CAD build for the part. Positions are in the model's coordinates, mm. A direction names the side the tool comes from. Give positions to 0.01 mm unless a question says otherwise; leave off trailing zeros. Write each loop counter-clockwise with the first axis right and the second up, starting at its lowest first coordinate (ties: lowest second). Pieces come first, ordered by that corner, then holes. Notation, with made-up numbers: (-12.5, 73) - (-7.5, 73) arc R21 cw to (-7.5, 83) - close; hole circle Ø2 at (41, -36.75). An arc over 180 degrees is marked (long way). Answer as a JSON object with one key per item and string values.
from build123d import *

# Parameters (mm, degrees)
SKETCH1_R               = 19.05
BASE_EXTRUDE_DEPTH      = 47.625
CUT_EXTRUDE1_DEPTH      = 20.05
CUT_EXTRUDE1_DEPTH_BACK = 20.05
CUT_EXTRUDE5_DEPTH      = 20.0500001
CUT_EXTRUDE5_DEPTH_BACK = 20.0500001
SKETCH11_R              = 4.7625
CUT_EXTRUDE6_DEPTH      = 20.0500001
CUT_EXTRUDE6_DEPTH_BACK = 20.0500001
SKETCH12_R              = 4.7625
CUT_EXTRUDE7_DEPTH      = 48.625000104
SCALE1_SCALE            = 0.65


with BuildPart() as part:
    # Sketch1 → Base-Extrude (new body)
    with BuildSketch(Plane(origin=(0, 0, 0), x_dir=(-1, 0, 0), z_dir=(0, 1, 0))):
        Circle(SKETCH1_R)
    extrude(amount=BASE_EXTRUDE_DEPTH)

    # Sketch2 → Cut-Extrude1 (cut, two sides)
    with BuildSketch(Plane.XY) as cut_extrude1_sk:
        with BuildLine():
            Line((-19.05, -131.979516723), (-19.05, 0))
            Line((-19.05, 0), (-19.05, 29.21))
            ThreePointArc((-19.05, 29.21), (-12.314807909, 26.420192091), (-9.525, 19.685))
            Line((-9.525, 19.685), (-9.525, 9.525))
            ThreePointArc((-9.525, 9.525), (0, 0), (9.525, 9.525))
            Line((9.525, 9.525), (9.525, 19.685))
            ThreePointArc((9.525, 19.685), (12.314807909, 26.420192091), (19.05, 29.21))
            Line((19.05, 29.21), (19.05, 0))
            Line((19.05, 0), (19.05, -131.979516723))
            Line((19.05, -131.979516723), (19.05, -395.938550169))
            Line((19.05, -395.938550169), (-19.05, -395.938550169))
            Line((-19.05, -395.938550169), (-19.05, -131.979516723))
        make_face()
    extrude(amount=CUT_EXTRUDE1_DEPTH, mode=Mode.SUBTRACT)
    extrude(cut_extrude1_sk.sketch, amount=-CUT_EXTRUDE1_DEPTH_BACK, mode=Mode.SUBTRACT)

    # Sketch8 → Cut-Extrude5 (cut, two sides)
    with BuildSketch(Plane(origin=(0, 0, 0), x_dir=(0, 0, -1), z_dir=(1, 0, 0))) as cut_extrude5_sk:
        Polygon((-10.16, -121.738350451), (-10.16, 0), (-10.16, 29.145238826), (10.16, 29.145238826), (10.16, 0), (10.16, -121.738350451), (10.16, -365.215051352), (-10.16, -365.215051352), align=None)
    extrude(amount=CUT_EXTRUDE5_DEPTH, mode=Mode.SUBTRACT)
    extrude(cut_extrude5_sk.sketch, amount=-CUT_EXTRUDE5_DEPTH_BACK, mode=Mode.SUBTRACT)

    # Sketch11 → Cut-Extrude6 (cut, two sides)
    with BuildSketch(Plane.XY) as cut_extrude6_sk:
        with Locations((0, 9.525)):
            Circle(SKETCH11_R)
    extrude(amount=CUT_EXTRUDE6_DEPTH, mode=Mode.SUBTRACT)
    extrude(cut_extrude6_sk.sketch, amount=-CUT_EXTRUDE6_DEPTH_BACK, mode=Mode.SUBTRACT)

    # Sketch12 → Cut-Extrude7 (cut, through all)
    with BuildSketch(Plane(origin=(0, 47.625, 0), x_dir=(-1, 0, 0), z_dir=(0, 1, 0))):
        Circle(SKETCH12_R)
    extrude(amount=-CUT_EXTRUDE7_DEPTH, mode=Mode.SUBTRACT)


with BuildPart() as part_1:
    # Scale1: scaled about (-0.00021981, 32.483233493, 0.000100002)
    add(part.part.scale(SCALE1_SCALE).moved(Location((-7.6933e-05, 11.369131723, 3.5001e-05))))


solid = part_1.part
(1) Saw through at C-C, the plane x = 0.5. Give the cut face in (y, z) (3 decimals), and give its area (3 significant figures).
Answer key:
{"outline": "(11.389, -12.372) - (14.505, -12.372) - (14.505, -6.604) - (11.389, -6.604) - close; (11.389, 6.604) - (14.505, 6.604) - (14.505, 12.372) - (11.389, 12.372) - close; (20.615, -12.372) - (42.325, -12.372) - (42.325, -3.055) - (30.314, -3.055) - (30.314, -6.604) - (20.615, -6.604) - close; (20.615, 6.604) - (30.314, 6.604) - (30.314, 3.055) - (42.325, 3.055) - (42.325, 12.372) - (20.615, 12.372) - close", "area": "372 mm²"}
(2) Saw through at D-D, the plane z = 1. Give the cut face in (x, y), and give its area (3 significant figures).
Answer key:
{"outline": "(-12.34, 30.36) arc R6.19 cw to (-11.66, 30.31) - (-2.93, 30.31) - (-2.93, 42.33) - (-12.34, 42.33) - close; (2.93, 30.31) - (11.66, 30.31) arc R6.19 cw to (12.34, 30.36) - (12.34, 42.33) - (2.93, 42.33) - close", "area": "226 mm²"}
(3) 3-axis set-ups, long thin cutter, end or side, ignore diameter. For faces 4 (the face through (0, 23, 6.604)), 5 (the face through (-6.191, 21, -9)), 6 (the face through (6.191, 21, -9)): which of +Z, -Z, +X, -X, +Y, -Y reach the whole face in a straight line?
Answer key:
{"face 4": "+X, -X, -Y", "face 5": "+Z, -Z, -X, -Y", "face 6": "+Z, -Z, +X, -Y"}
(4) Pull direction Z, two halves, no side cores. Call faces 1 (the face through (1.4, 14.8, 9.5)), 2 (the face through (2.68, 33.51, -12.09)), 3 (the face through (0, 23, -6.604)): pulls with the +Z half, pulls with the -Z half, needs draft (parallel to the pull), parting line crosses it, or undercut.
Answer key:
{"face 1": "needs draft", "face 2": "parting line crosses it", "face 3": "undercut"}
(5) Flat gauge pins, fed straight in: P1, Ø2, axis at y = 20.5, z = -9.5, coming from the +X side; P2, Ø4, axis at x = 1, z = -1, coming from the -Y side; P3, Ø6, axis at y = 39, z = 4.5, coming from the -X side. Where does each tip first touch, or does it go through?
Answer key:
{"P1": "stops at x = 6.19", "P2": "stops at y = 30.31", "P3": "stops at x = -12.29"}
(6) Saw through at B-B, the plane z = 8. Give the cut face in (x, y), and give its area (3 significant figures).
Answer key:
{"outline": "(-9.45, 29.62) arc R6.19 cw to (-6.19, 24.16) - (-6.19, 17.56) arc R6.19 ccw to (6.19, 17.56) - (6.19, 24.16) arc R6.19 cw to (9.45, 29.62) - (9.45, 42.33) - (-9.45, 42.33) - close; hole circle Ø6.19 at (0, 17.56)", "area": "430 mm²"}
(7) Probe L1, parallel to Y at x = 5.5, z = 0.5; L2, parallel to Z at x = -4, y = 17; L3, parallel to X at y = 35.5, z = 2.25. List the from-to ranges inside material, lowest first. Write a range as [from, to].
Answer key:
{"L1": "y = [30.31, 42.33]", "L2": "z = [-11.72, -6.6], [6.6, 11.72]", "L3": "x = [-12.18, -2.13], [2.13, 12.18]"}
(8) Saw through at A-A, the plane y = 22. Give the cut face in (x, z) (1 decimal).
Answer key:
{"outline": "(-6.2, -10.7) arc R12.4 ccw to (6.2, -10.7) - (6.2, -6.6) - (-6.2, -6.6) - close; (-6.2, 6.6) - (6.2, 6.6) - (6.2, 10.7) arc R12.4 ccw to (-6.2, 10.7) - close"}
